Verification items for the finished model (mm, model axes). A direction names the side the tool comes from. Give positions to 0.01 mm unless a question says otherwise; leave off trailing zeros. Write each loop counter-clockwise with the first axis right and the second up, starting at its lowest first coordinate (ties: lowest second). Pieces come first, ordered by that corner, then holes. Notation, with made-up numbers: (75.5, 24.5) -> (92.5, 24.5) arc R22 ccw to (92.5, 30.5) -> close; hole circle Ø9 at (78, 41.25). An arc over 180 degrees is marked (long way). Answer as CSV lines item,"result". Start each with the question number.
1) Sectioned sample at B-B on z = -17. Record the cut outline in (x, y) (3 decimals).
2) Mould release check, pull along X, two halves, no side actions. Record for faces 6 (the flat face through (-26.28, -21.75, -8.87)), 7 (the cylindrical face through (1.811, 82.648, -40.648)), 8 (the flat face through (-19.23, 2.41, -18.14)): released by +X, released by -X, zero draft, split by the parting line, or undercut.
3) Material ranges on L1, parallel to X at y = -24, z = -11; L2, parallel to Y at x = -43, z = -10; L3, parallel to Z at x = 42, y = 27, recorded low to high.
4) Gauge pin test, flat ends, axial feed: pin 1 Ø8.5 at (x, z) = (-20, -3.5) entering from -Y; pin 2 Ø10.5 at (x, y) = (-32, -22) entering from +Z; pin 3 Ø2 at (x, z) = (35.5, -19) entering from +Y; pin 4 Ø10 at (x, z) = (-30, -31.5) entering from +Y. Record the tip position at first contact, or that the pin passes through.
5) Sectioned sample at C-C on y = -15.5. Record the cut outline in (x, z), and give its area (3 significant figures).
6) Sectioned sample at A-A on x = -43.18. Record the cut outline in (y, z).
7) Sectioned sample at D-D on z = 3. Record the cut outline in (x, y) (3 decimals).
8) Tool access check on faces 1 (the cylindrical face through (1.811, 74.134, -37.614)), 2 (the flat face through (-26.32, -26.58, -8.87)), 3 (the flat face through (-38, -6.35, -25)), 4 (the cylindrical face through (39.6, -6.69, -17.42)), 5 (the cylindrical face through (-43.36, -21.47, -44.66)). Record the directions out of +Z, -Z, +X, -X, +Y, -Y that give a thin tool (end or side, any length) a straight path to the whole face; none if there is none.
```python
from build123d import *

# Parameters (mm, degrees)
BOSS_EXTRUDE1_DEPTH  = 8.889999999999999
BOSS_EXTRUDE2_DEPTH  = 38.1
SKETCH15_W           = 41.9077442661452
SKETCH15_H           = 43.17111295633907
CUT_EXTRUDE2_DEPTH   = 97.53600000000003
BOSS_EXTRUDE5_START  = 12.7
BOSS_EXTRUDE5_DEPTH  = 12.7
BOSS_EXTRUDE6_DEPTH  = 5.08
BOSS_EXTRUDE7_DEPTH  = 5.08
BOSS_EXTRUDE9_START  = -25.4
BOSS_EXTRUDE9_DEPTH  = 5.08
SKETCH20_R           = 2.6670000000000025
SKETCH20_R_2         = 2.6669999999999994
CUT_EXTRUDE3_DEPTH   = 79.56569416736545
BOSS_EXTRUDE10_START = 43.18
BOSS_EXTRUDE10_DEPTH = 43.18
FILLET2_R            = 2.54
CUT_EXTRUDE4_DEPTH   = 2.54
SKETCH22_W           = 21.77675569209209
SKETCH22_H           = 4.484390369282897
CUT_EXTRUDE5_DEPTH   = 73.97805012467812
BOSS_EXTRUDE11_START = 7.62
SKETCH23_R           = 2.6669999999999994
SKETCH23_R_2         = 2.6670000000000025
BOSS_EXTRUDE11_DEPTH = 7.62
FILLET3_R            = 5.08
BOSS_EXTRUDE12_START = -52.07
BOSS_EXTRUDE12_DEPTH = 52.07
FILLET4_R            = 1.27
FILLET5_R            = 20.32
BOSS_EXTRUDE13_DEPTH = 104.14
FILLET6_R            = 0.508
FILLET7_R            = 7.619999999999999
FILLET8_R            = 25.4
FILLET9_R            = 1.27


with BuildPart() as part:
    # Sketch1 → Boss-Extrude1 (new body)
    with BuildSketch(Plane.XY):
        with BuildLine():
            Line((-31.75, -11.43), (-11.429999999999998, -11.429999999999993))
            Line((-11.429999999999998, -11.429999999999993), (-11.43, 0))
            ThreePointArc((-11.43, 0), (7e-16, 11.43), (11.43, 0))
            Line((11.43, 0), (11.429999999999998, -11.42999999999999))
            Line((11.429999999999998, -11.42999999999999), (31.75, -11.429999999999993))
            Line((31.75, -11.429999999999993), (11.77180119767475, 10.650836660207654))
            ThreePointArc((11.77180119767475, 10.650836660207654), (9.7e-16, 15.875), (-11.771801197674753, 10.65083666020765))
            Line((-11.771801197674753, 10.65083666020765), (-31.75, -11.43))
        make_face()
    extrude(amount=BOSS_EXTRUDE1_DEPTH)

    # Sketch11 → Boss-Extrude2 (add)
    with BuildSketch(Plane(origin=(0, 0, 0), x_dir=(-1, 0, 0), z_dir=(0, 0, -1))):
        Polygon((27.153740742364707, -6.350000000000002), (31.75, -11.43), (11.429999999999998, -11.429999999999993), (11.429999999999996, -6.349999999999992), align=None)
    extrude(amount=BOSS_EXTRUDE2_DEPTH)

    # Sketch15 → Cut-Extrude2 (cut)
    with BuildSketch(Plane.XY.offset(8.889999999999999)):
        with Locations((20.9538721330726, 0.9898585075243087)):
            Rectangle(SKETCH15_W, SKETCH15_H)
    extrude(amount=-CUT_EXTRUDE2_DEPTH, mode=Mode.SUBTRACT)

    # Sketch16 → Boss-Extrude5 (add)
    with BuildSketch(Plane(origin=(0, 0, 0), x_dir=(-1, 0, 0), z_dir=(0, 0, -1)).offset(BOSS_EXTRUDE5_START)):
        with BuildLine():
            Line((11.771801197674753, 10.65083666020765), (27.153740742364707, -6.350000000000003))
            Line((27.153740742364707, -6.350000000000003), (11.429999999999996, -6.349999999999992))
            Line((11.429999999999996, -6.349999999999992), (11.43, -3.9e-15))
            ThreePointArc((11.43, -3.9e-15), (8.082230508962239, 8.082230508962237), (0, 11.43))
            Line((0, 11.43), (0, 15.875))
            ThreePointArc((0, 15.875), (6.4394717570311455, 14.510300771879203), (11.771801197674753, 10.65083666020765))
        make_face()
    extrude(amount=-BOSS_EXTRUDE5_DEPTH)

    # Sketch18 → Boss-Extrude6 (add)
    with BuildSketch(Plane(origin=(4.2e-15, -6.3499999999999845, 0), x_dir=(1, 2.8e-16, 0), z_dir=(-2.8e-16, 1, 0))):
        Polygon((-11.430000000000001, 12.70000000000001), (-49.53, 12.700000000000006), (-49.53, 38.099999999999994), (-11.43, 38.1), align=None)
    extrude(amount=-BOSS_EXTRUDE6_DEPTH)

    # Sketch19 → Boss-Extrude7 (add)
    with BuildSketch(Plane(origin=(0, 0, -38.1), x_dir=(-1, 0, 0), z_dir=(0, 0, -1))):
        Polygon((11.429999999999998, -6.349999999999998), (49.53, -6.349999999999991), (49.53, -31.749999999999986), (11.43, -31.75), align=None)
    extrude(amount=BOSS_EXTRUDE7_DEPTH)

    # Sketch19<3> → Boss-Extrude9 (add)
    with BuildSketch(Plane(origin=(0, 0, -38.1), x_dir=(-1, 0, 0), z_dir=(0, 0, -1)).offset(BOSS_EXTRUDE9_START)):
        Polygon((11.429999999999998, -6.349999999999998), (49.53, -6.349999999999991), (49.53, -31.749999999999986), (11.43, -31.75), align=None)
    extrude(amount=-BOSS_EXTRUDE9_DEPTH)

    # Sketch20 → Cut-Extrude3 (cut, through all)
    with BuildSketch(Plane(origin=(0, 0, -43.18), x_dir=(-1, 0, 0), z_dir=(0, 0, -1))):
        with Locations(Location((30.48, -24.129999999999992, 0), (0, 0, 180))):
            Circle(SKETCH20_R)
        with Locations(Location((17.78, -24.129999999999992, 0), (0, 0, 180))):
            Circle(SKETCH20_R_2)
        with Locations(Location((43.17999999999999, -24.129999999999992, 0), (0, 0, 180))):
            Circle(SKETCH20_R)
    extrude(amount=-CUT_EXTRUDE3_DEPTH, mode=Mode.SUBTRACT)

    # Sketch16<2> → Boss-Extrude10 (add)
    with BuildSketch(Plane(origin=(0, 0, 0), x_dir=(-1, 0, 0), z_dir=(0, 0, -1)).offset(BOSS_EXTRUDE10_START)):
        with BuildLine():
            Line((11.771801197674753, 10.65083666020765), (27.153740742364707, -6.350000000000003))
            Line((27.153740742364707, -6.350000000000003), (11.429999999999996, -6.349999999999992))
            Line((11.429999999999996, -6.349999999999992), (11.43, -3.9e-15))
            ThreePointArc((11.43, -3.9e-15), (8.082230508962239, 8.082230508962237), (0, 11.43))
            Line((0, 11.43), (0, 15.875))
            ThreePointArc((0, 15.875), (6.4394717570311455, 14.510300771879203), (11.771801197674753, 10.65083666020765))
        make_face()
    extrude(amount=-BOSS_EXTRUDE10_DEPTH)

    # Fillet2
    fillet2_edges = [part.edges().sort_by_distance(p)[0] for p in [
        (-11.43, -31.75, -40.64),
        (-49.53, -31.749999999999986, -40.64),
        (-11.43, -31.75, -10.160000000000004),
        (-27.153740742364704, -6.35, -25.400000000000002),
        (-49.53, -31.749999999999986, -10.160000000000004),
        (-49.53, -6.349999999999991, -25.400000000000002),
    ]]
    fillet(fillet2_edges, radius=FILLET2_R)

    # Sketch21 → Cut-Extrude4 (cut)
    with BuildSketch(Plane.XY.offset(-7.620000000000012)):
        Polygon((-27.69370760089086, -19.303999999999988), (-33.26629239910914, -19.303999999999988), (-36.052584798218284, -24.129999999999992), (-33.26629239910914, -28.955999999999996), (-27.693707600890868, -28.955999999999996), (-24.907415201781728, -24.129999999999985), align=None)
        Polygon((-40.393707600890856, -19.303999999999988), (-45.96629239910914, -19.303999999999988), (-48.75258479821828, -24.129999999999992), (-45.96629239910914, -28.955999999999996), (-40.39370760089086, -28.955999999999996), (-37.60741520178173, -24.129999999999985), align=None)
        Polygon((-14.99370760089086, -19.303999999999988), (-20.56629239910914, -19.303999999999988), (-23.352584798218277, -24.129999999999992), (-20.56629239910914, -28.955999999999996), (-14.993707600890867, -28.955999999999996), (-12.20741520178173, -24.129999999999985), align=None)
    extrude(amount=-CUT_EXTRUDE4_DEPTH, mode=Mode.SUBTRACT)

    # Sketch22 → Cut-Extrude5 (cut, through all)
    with BuildSketch(Plane.ZY.offset(49.53)):
        Polygon((-38.354, -11.42999999999998), (-12.446000000000005, -11.42999999999998), (-12.446000000000002, -35.87938903250851), (-38.354, -35.87938903250852), align=None)
        with Locations((3.268377846046038, -13.16419518464144)):
            Rectangle(SKETCH22_W, SKETCH22_H)
    extrude(amount=-CUT_EXTRUDE5_DEPTH, mode=Mode.SUBTRACT)

    # Sketch23 → Boss-Extrude11 (add)
    with BuildSketch(Plane(origin=(0, 0, -43.18), x_dir=(-1, 0, 0), z_dir=(0, 0, -1)).offset(BOSS_EXTRUDE11_START)):
        with BuildLine():
            Line((46.990000000000016, -31.749999999999993), (-54.60999999999998, -31.75))
            Line((-54.60999999999998, -31.75), (-54.60999999999998, 59.690000000000005))
            Line((-54.60999999999998, 59.690000000000005), (49.52999999999999, 59.690000000000005))
            Line((49.52999999999999, 59.690000000000005), (49.53, -29.209999999999987))
            ThreePointArc((49.53, -29.209999999999987), (48.786051224213836, -31.006051224213813), (46.990000000000016, -31.749999999999993))
        make_face()
        with Locations((17.78, -24.129999999999992)):
            Circle(SKETCH23_R, mode=Mode.SUBTRACT)
        with Locations((30.48, -24.129999999999992)):
            Circle(SKETCH23_R_2, mode=Mode.SUBTRACT)
        with Locations((43.17999999999999, -24.129999999999992)):
            Circle(SKETCH23_R_2, mode=Mode.SUBTRACT)
    extrude(amount=-BOSS_EXTRUDE11_DEPTH)

    # Fillet3
    fillet3_edges = [part.edges().sort_by_distance(p)[0] for p in [
        (54.60999999999998, -31.75, -46.989999999999995),
    ]]
    fillet(fillet3_edges, radius=FILLET3_R)

    # Sketch24 → Boss-Extrude12 (add)
    with BuildSketch(Plane.XY.offset(8.889999999999999).offset(BOSS_EXTRUDE12_START)):
        with BuildLine():
            Line((5.067787914863957, 10.245117161358323), (39.587974363799084, -6.83043023839146))
            Line((39.587974363799084, -6.83043023839146), (58.38762081865667, -11.17067060922455))
            Line((58.38762081865667, -11.17067060922455), (7.03859432619994, 14.229329390775446))
            ThreePointArc((7.03859432619994, 14.229329390775446), (3.6142095208661993, 15.458108375195204), (0, 15.875))
            Line((0, 15.875), (-7e-16, 11.43))
            ThreePointArc((-7e-16, 11.43), (2.6022308550236635, 11.129838030140547), (5.067787914863957, 10.245117161358323))
        make_face()
    extrude(amount=BOSS_EXTRUDE12_DEPTH)

    # Fillet4
    # the kernel refuses this fillet: 1.27 mm, written as the material it takes off along each edge
    with BuildSketch(Plane(origin=(58.38762081865667, -11.17067060922455, -43.18), x_dir=(-0.8963357096551464, 0.4433760205480277, 0), z_dir=(0, 0, 1))) as fillet4_piece_1:
        with BuildLine():
            CenterArc((FILLET4_R * 8.56452358423, FILLET4_R), FILLET4_R, 103.31948375813553, 166.68051624186455)
            Line((FILLET4_R * 8.3341429253, FILLET4_R * 1.97310058678), (0, 0))
            Line((0, 0), (FILLET4_R * 8.56452358423, -1.2e-16))
        make_face()
    extrude(amount=79.2623623799331, mode=Mode.SUBTRACT)

    # Fillet5
    fillet5_edges = [part.edges().sort_by_distance(p)[0] for p in [
        (39.587974363799084, -6.83043023839146, -17.145),
    ]]
    fillet(fillet5_edges, radius=FILLET5_R)

    # Sketch25 → Boss-Extrude13 (add)
    with BuildSketch(Plane.ZY.offset(49.53)):
        with BuildLine():
            Line((-29.028140773868504, 83.30403252851806), (-21.7408262217295, 95.69350349416987))
            ThreePointArc((-21.7408262217295, 95.69350349416987), (-41.35451230486861, 81.7952335654154), (-50.800000000000004, 59.69000000000002))
            Line((-50.800000000000004, 59.69000000000002), (-43.18, 59.69000000000002))
            ThreePointArc((-43.18, 59.69000000000002), (-38.40361060567099, 72.87512775034637), (-29.028140773868504, 83.30403252851806))
        make_face()
    extrude(amount=-BOSS_EXTRUDE13_DEPTH)

    # Fillet6
    fillet6_edges = [part.edges().sort_by_distance(p)[0] for p in [
        (2.5399999999999707, 95.69350349416987, -21.7408262217295),
    ]]
    fillet(fillet6_edges, radius=FILLET6_R)

    # Fillet7
    fillet7_edges = [part.edges().sort_by_distance(p)[0] for p in [
        (2.539999999999978, 83.30403252851806, -29.028140773868504),
    ]]
    fillet(fillet7_edges, radius=FILLET7_R)

    # Fillet8
    fillet8_edges = [part.edges().sort_by_distance(p)[0] for p in [
        (2.539999999999999, 59.690000000000005, -50.8),
        (2.539999999999999, 59.690000000000005, -43.18),
    ]]
    fillet(fillet8_edges, radius=FILLET8_R)

    # Fillet9
    fillet9_edges = [part.edges().sort_by_distance(p)[0] for p in [
        (-21.531087635955615, -0.13558166989617781, 8.889999999999999),
        (-11.43, -5.460999999999997, 8.889999999999999),
        (-2.9668526046512183, 15.59530091477155, 8.889999999999999),
        (21.264567959032345, 2.2333155514035123, 8.889999999999999),
        (27.83841048622558, 3.940617675038018, 8.889999999999999),
        (49.271107203403254, -7.9137111445449655, 8.89),
        (44.84459728880309, -8.044017264516304, 8.889999999999999),
        (39.63441669939814, -6.700434090326565, 8.89),
        (-6.029928860820195, 9.710039028420407, 8.889999999999999),
    ]]
    fillet(fillet9_edges, radius=FILLET9_R)


solid = part.part
```
Ans:
1,outline,"(-49.53, -11.43) -> (-11.43, -11.43) -> (-11.43, 0) arc R11.43 cw to (5.068, 10.245) -> (37.461, -5.778) arc R20.32 ccw to (41.9, -7.364) -> (47.789, -8.724) arc R1.27 ccw to (48.638, -6.348) -> (7.039, 14.229) arc R15.875 ccw to (-11.772, 10.651) -> (-26.397, -5.514) arc R2.54 cw to (-28.281, -6.35) -> (-46.99, -6.35) arc R2.54 ccw to (-49.53, -8.89) -> close"
2,face 6,"undercut"
2,face 7,"zero draft"
2,face 8,"released by -X"
3,L1,"x = -49.53 to -45.84, -40.52 to -33.14, -27.82 to -20.44, -15.12 to -11.43"
3,L2,"y = -31.75 to -28.96, -19.3 to -6.35"
3,L3,"z = -50.8 to -43.18"
4,pin 1,"stops at y = -31.75"
4,pin 2,"stops at z = -7.62"
4,pin 3,"stops at y = 0.65"
4,pin 4,"stops at y = 93.68"
5,outline,"(-49.53, -50.8) -> (54.61, -50.8) -> (54.61, -43.18) -> (-11.43, -43.18) -> (-11.43, -38.35) -> (-49.53, -38.35) -> close; (-49.53, -12.45) -> (-11.43, -12.45) -> (-11.43, -7.62) -> (-49.53, -7.62) -> close"
5,area,"1,160 mm²"
6,outline,"(-31.75, -50.8) -> (-26.8, -50.8) -> (-26.8, -38.35) -> (-31.75, -38.35) -> close; (-31.75, -12.45) -> (-26.8, -12.45) -> (-26.8, -10.16) -> (-28.96, -10.16) -> (-28.96, -7.62) -> (-31.75, -7.62) -> close; (-21.46, -50.8) -> (57.71, -50.8) arc R25.4 ccw to (62.69, -50.31) arc R44.22 ccw to (95.19, -23.09) arc R0.51 ccw to (94.46, -22.47) -> (84.55, -28.3) arc R7.62 ccw to (82.5, -30.06) arc R36.68 cw to (64.17, -42.19) arc R25.4 cw to (57.14, -43.18) -> (-6.35, -43.18) -> (-6.35, -7.62) -> (-19.3, -7.62) -> (-19.3, -10.16) -> (-21.46, -10.16) -> (-21.46, -12.45) -> (-11.43, -12.45) -> (-11.43, -38.35) -> (-21.46, -38.35) -> close"
7,outline,"(-31.29, -10.922) -> (-11.43, -10.922) -> (-11.43, 0) arc R11.43 cw to (5.068, 10.245) -> (37.461, -5.778) arc R20.32 ccw to (41.9, -7.364) -> (47.789, -8.724) arc R1.27 ccw to (48.638, -6.348) -> (7.039, 14.229) arc R15.875 ccw to (-11.772, 10.651) -> close"
8,face 1,"+Z, +X, -X"
8,face 2,"+Z"
8,face 3,"+Z, -X"
8,face 4,"+Z, -Y"
8,face 5,"+Z, -Z"
